```python
from build123d import *

# Parameters (mm, degrees)
SKETCH1_W               = 43.25
SKETCH1_H               = 31.5
BOSS_EXTRUDE1_DEPTH     = 23
CUT_EXTRUDE1_DEPTH      = 20
CUT_EXTRUDE2_DEPTH      = 55.663882043
CUT_EXTRUDE2_DEPTH_BACK = 55.663882043
SKETCH3_R               = 0.8


with BuildPart() as part:
    # Sketch1 → Boss-Extrude1 (new body)
    with BuildSketch(Plane(origin=(0, 0, 0), x_dir=(1, 0, 0), z_dir=(0, 1, 0))):
        with Locations((21.625, 15.75)):
            Rectangle(SKETCH1_W, SKETCH1_H)
    extrude(amount=BOSS_EXTRUDE1_DEPTH)

    # Sketch2 → Cut-Extrude1 (cut)
    with BuildSketch(Plane(origin=(0, 23, 0), x_dir=(1, 0, 0), z_dir=(0, 1, 0))):
        Polygon((38.3, 28.5), (5.8, 28.5), (5.8, 25.5), (3.8, 25.5), (3.8, 6), (5.8, 6), (5.8, 3), (38.3, 3), (38.3, 8.2), (39.45, 8.2), (39.45, 23.3), (38.3, 23.3), align=None)
    extrude(amount=-CUT_EXTRUDE1_DEPTH, mode=Mode.SUBTRACT)

    # Sketch3 → Cut-Extrude2 (cut, two sides: drawn at the far end of the back side and taken through both)
    with BuildSketch(Plane.ZY.offset(-38.3).offset(-CUT_EXTRUDE2_DEPTH_BACK)):
        with Locations((-26.55, 9)):
            Circle(SKETCH3_R)
        with Locations((-6.05, 9)):
            Circle(SKETCH3_R)
    extrude(amount=CUT_EXTRUDE2_DEPTH + CUT_EXTRUDE2_DEPTH_BACK, mode=Mode.SUBTRACT)


solid = part.part
```
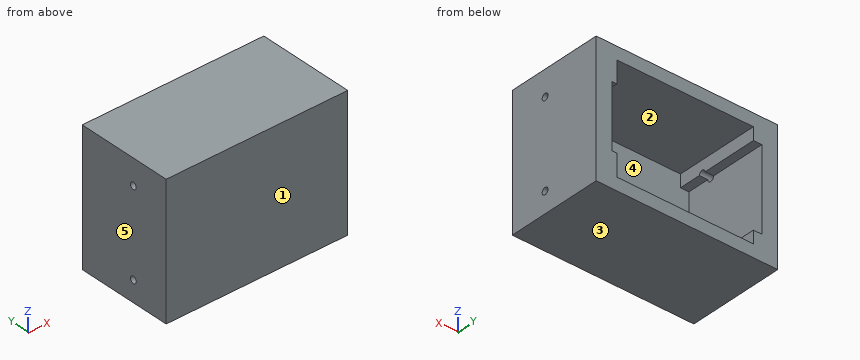
Can you work these out from the model? Positions are in its coordinate system, mm. Face numbers are marked on the shaded views. A direction names the side the tool comes from. Coordinates: 2 decimals unless noted, no trailing zeros. Loops run counter-clockwise (first coordinate to the right, second up) from the corner with the lowest first, then second, coordinate; pieces in that order, holes last.
Item 1: If we mould it in two halves opening along Z, with no side actions, what happens to the marked faces 3, 4 and 5? For each: released by +Z, released by -Z, zero draft, split by the parting line, or undercut.
Answers below:
face 3: released by -Z
face 4: undercut
face 5: zero draft
Item 2: Suppose I cut it at A-A (y = 9). State how many separate pieces and enclosed holes the cut face has, then the cut area to 3 significant figures.
Answers below:
separate pieces: 4
enclosed holes: 0
area: 445 mm2
Item 3: I'm going to push flat-ended pins straight in: pin 1 (4 mm diameter, centred on x = 35, z = -12, fed in from +Y); pin 2 (1.4 mm diameter, centred on y = 9, z = -26.55, fed in from -X). Where does each tip first touch, or does it pass through?
Answers below:
pin 1: stops at y = 3
pin 2: passes through
Item 4: Suppose I cut it at D-D (x = 20.5). Please give me the cut outline in (y, z).
Answers below:
outline: (0, -31.5) - (23, -31.5) - (23, -28.5) - (3, -28.5) - (3, -3) - (23, -3) - (23, 0) - (0, 0) - close
Item 5: Suppose I cut it at B-B (z = -26.55). Please give me the cut outline in (x, y).
Answers below:
outline: (0, 0) - (43.25, 0) - (43.25, 8.2) - (38.3, 8.2) - (38.3, 3) - (5.8, 3) - (5.8, 8.2) - (0, 8.2) - close; (0, 9.8) - (5.8, 9.8) - (5.8, 23) - (0, 23) - close; (38.3, 9.8) - (43.25, 9.8) - (43.25, 23) - (38.3, 23) - close
Item 6: Suppose I cut it at C-C (y = 17.75). Please give me the cut outline in (x, z), then the cut area to 3 significant figures.
Answers below:
outline: (0, -31.5) - (43.25, -31.5) - (43.25, 0) - (0, 0) - close; hole (3.8, -25.5) - (5.8, -25.5) - (5.8, -28.5) - (38.3, -28.5) - (38.3, -23.3) - (39.45, -23.3) - (39.45, -8.2) - (38.3, -8.2) - (38.3, -3) - (5.8, -3) - (5.8, -6) - (3.8, -6) - close
area: 477 mm2
Item 7: Please list where these lines run through material, in increasing order: L1, parallel to Z at x = 3.9, y = 9; L2, parallel to Z at x = 41.95, y = 9; L3, parallel to X at y = 12.5, z = -12.
Answers below:
L1: z = -31.5 to -27.35, -25.75 to -25.5, -5.25 to 0
L2: z = -31.5 to -27.35, -25.75 to -6.85, -5.25 to 0
L3: x = 0 to 3.8, 39.45 to 43.25
Item 8: Which directions (+Z, -Z, +X, -X, +Y, -Y) give clear straight access to the entire face, cutting with the end or side of a thin tool? Please do the marked faces 1 and 2.
Answers below:
face 1: +Z, -Z, +X, -X, -Y
face 2: +Y
